from build123d import *

# Parameters (mm, degrees)
F0_R          = 12.5
F1_DEPTH      = 90
F1_DEPTH_BACK = 90
F2_R          = 9.5
F3_DEPTH      = 14
F4_SIZE       = 2
F5_R          = 9.5
F6_DEPTH      = 14
F7_SIZE       = 2


with BuildPart() as f1:
    # F0 (on Front) → F1 (new body, two sides)
    with BuildSketch(Plane.XZ) as f1_sk:
        Circle(F0_R)
    extrude(amount=F1_DEPTH)
    extrude(f1_sk.sketch, amount=-F1_DEPTH_BACK)

    # F2 (on face) → F3 (cut)
    with BuildSketch(Plane.XZ.offset(90)):
        Circle(F2_R)
    extrude(amount=-F3_DEPTH, mode=Mode.SUBTRACT)

    # F4
    f4_edges = [f1.edges().sort_by_distance(p)[0] for p in [
        (-12.5, -90, 0),
    ]]
    chamfer(f4_edges, length=F4_SIZE)

    # F5 (on face) → F6 (cut)
    with BuildSketch(Plane(origin=(0, 90, 0), x_dir=(-1, 0, 0), z_dir=(0, 1, 0))):
        Circle(F5_R)
    extrude(amount=-F6_DEPTH, mode=Mode.SUBTRACT)

    # F7
    f7_edges = [f1.edges().sort_by_distance(p)[0] for p in [
        (-12.5, 90, 0),
    ]]
    chamfer(f7_edges, length=F7_SIZE)


solid = f1.part
The listing builds one solid part. Answer for the finished solid, in the listing's coordinates (mm). A direction names the side the tool comes from. Coordinates: 2 decimals unless noted, no trailing zeros. Loops run counter-clockwise (first coordinate to the right, second up) from the corner with the lowest first, then second, coordinate; pieces in that order, holes last. Notation, with made-up numbers: (0.25, 53) -> (43.25, 53) arc R27 cw to (43.25, 80) -> close; hole circle Ø2 at (-13.75, 15.25). An arc over 180 degrees is marked (long way). Answer in a Markdown table with one row per item. Add a question column.
1. For faces 1 (the flat face through (0, 76, 0)), 2 (the flat face through (0, -76, 0)), 3 (the flat face through (-5, -90, -9)), determine the directions among +Z, -Z, +X, -X, +Y, -Y from which every point of the face is accessible in a straight line to the end or side of a thin tool.
2. Determine the mould class of faces 4 (the cylindrical face through (11.923, -1.232, 3.755)), 5 (the cylindrical face through (4.38, -83.1, -8.43)), 6 (the flat face through (-5, 90, -9)) for opening direction X: +X half, -X half, draft (parallel to the pull), parting line (faces both ways), or undercut.
3. Consider line 1 (Z direction, x = 0, y = -81.5); line 2 (Y direction, x = -3.5, z = -5.75); line 3 (Z direction, x = -8.25, y = 79.5). Determine where each line is inside the solid, lowest interval first. Write a range as [from, to].
4. The part is cut by section B-B, the plane z = 0. Write down the section's boundary in (x, y), then the cut area to 3 significant figures.
5. The part is cut by section A-A, the plane x = 0. Write down the section's boundary in (y, z).
6. Flat-ended cylindrical pins translate along their axes: P1, Ø1.5, axis at y = -17.5, z = 4.5, coming from the +X side; P2, Ø1.5, axis at y = -39.5, z = -2, coming from the +X side; P3, Ø3, axis at x = 1.5, y = 51.5, coming from the -Z side; P4, Ø9.5, axis at x = 1.5, z = 1.5, coming from the -Y side. Find the tip coordinate at first contact, or state that the pin passes through.
7. The part is cut by section C-C, the plane y = -30.5. Write down the section's boundary in (x, z), then the cut area to 3 significant figures.
Answer below:
| question | item | result |
|---|---|---|
| 1 | face 1 | +Y |
| 1 | face 2 | -Y |
| 1 | face 3 | +Z, -Z, +X, -X, -Y |
| 2 | face 4 | parting line |
| 2 | face 5 | undercut |
| 2 | face 6 | draft |
| 3 | line 1 | [-12.5, -9.5], [9.5, 12.5] |
| 3 | line 2 | [-76, 76] |
| 3 | line 3 | [-9.39, -4.71], [4.71, 9.39] |
| 4 | outline | (-12.5, -88) -> (-10.5, -90) -> (-9.5, -90) -> (-9.5, -76) -> (9.5, -76) -> (9.5, -90) -> (10.5, -90) -> (12.5, -88) -> (12.5, 88) -> (10.5, 90) -> (9.5, 90) -> (9.5, 76) -> (-9.5, 76) -> (-9.5, 90) -> (-10.5, 90) -> (-12.5, 88) -> close |
| 4 | area | 3,960 mm2 |
| 5 | outline | (-90, -10.5) -> (-88, -12.5) -> (88, -12.5) -> (90, -10.5) -> (90, -9.5) -> (76, -9.5) -> (76, 9.5) -> (90, 9.5) -> (90, 10.5) -> (88, 12.5) -> (-88, 12.5) -> (-90, 10.5) -> (-90, 9.5) -> (-76, 9.5) -> (-76, -9.5) -> (-90, -9.5) -> close |
| 6 | P1 | x = 11.92 |
| 6 | P2 | x = 12.44 |
| 6 | P3 | z = -12.5 |
| 6 | P4 | y = -76 |
| 7 | outline | circle Ø25 at (0, 0) |
| 7 | area | 491 mm2 |
